```python
from build123d import *

# Parameters (mm, degrees)
SKETCH2_W           = 60
SKETCH2_H           = 32.5
BOSS_EXTRUDE1_DEPTH = 3
SKETCH3_W           = 8
SKETCH3_H           = 4
BOSS_EXTRUDE2_DEPTH = 13
FILLET1_R           = 3
SKETCH4_R           = 2.5
CUT_EXTRUDE1_DEPTH  = 13
SKETCH5_R           = 2.5
CUT_EXTRUDE2_DEPTH  = 13
FILLET2_R           = 3
BOSS_EXTRUDE3_DEPTH = 6.5
FILLET3_R           = 2
SKETCH7_W           = 40
SKETCH7_H           = 10
BOSS_EXTRUDE4_DEPTH = 30
CUT_EXTRUDE3_DEPTH  = 30
FILLET5_R           = 3
SKETCH9_R           = 1
CUT_EXTRUDE4_DEPTH  = 5
FILLET6_R           = 3
FILLET7_R           = 3
FILLET8_R           = 3


with BuildPart() as part:
    # Sketch2 → Boss-Extrude1 (new body)
    with BuildSketch(Plane.XY):
        with Locations((-25.634473236, 6.404480792)):
            Rectangle(SKETCH2_W, SKETCH2_H)
    extrude(amount=BOSS_EXTRUDE1_DEPTH)

    # Sketch3 → Boss-Extrude2 (add)
    with BuildSketch(Plane.XY.offset(3)):
        with Locations((0.365526764, 20.654480792)):
            Rectangle(SKETCH3_W, SKETCH3_H)
        with Locations((0.365526764, -7.845519208)):
            Rectangle(SKETCH3_W, SKETCH3_H)
        with Locations((-51.634473236, 20.654480792)):
            Rectangle(SKETCH3_W, SKETCH3_H)
        with Locations((-51.634473236, -7.845519208)):
            Rectangle(SKETCH3_W, SKETCH3_H)
    extrude(amount=BOSS_EXTRUDE2_DEPTH)

    # Fillet1
    fillet1_edges = [part.edges().sort_by_distance(p)[0] for p in [
        (4.365526764, 20.654480792, 16),
        (-3.634473236, 20.654480792, 16),
        (4.365526764, -7.845519208, 16),
        (-3.634473236, -7.845519208, 16),
        (-55.634473236, 20.654480792, 16),
        (-47.634473236, 20.654480792, 16),
        (-55.634473236, -7.845519208, 16),
        (-47.634473236, -7.845519208, 16),
    ]]
    fillet(fillet1_edges, radius=FILLET1_R)

    # Sketch4 → Cut-Extrude1 (cut)
    with BuildSketch(Plane(origin=(0, 22.654480792, 0), x_dir=(1, 0, 0), z_dir=(0, 1, 0))):
        with Locations(Location((0.365526764, -12, 0), (0, 0, 270))):
            Circle(SKETCH4_R)
        with Locations(Location((-51.634473236, -12, 0), (0, 0, 270))):
            Circle(SKETCH4_R)
    extrude(amount=-CUT_EXTRUDE1_DEPTH, mode=Mode.SUBTRACT)

    # Sketch5 → Cut-Extrude2 (cut)
    with BuildSketch(Plane(origin=(0, -5.845519208, 0), x_dir=(1, 0, 0), z_dir=(0, 1, 0))):
        with Locations(Location((-51.634473236, -12, 0), (0, 0, 270))):
            Circle(SKETCH5_R)
        with Locations(Location((0.365526764, -12, 0), (0, 0, 270))):
            Circle(SKETCH5_R)
    extrude(amount=-CUT_EXTRUDE2_DEPTH, mode=Mode.SUBTRACT)

    # Fillet2
    fillet2_edges = [part.edges().sort_by_distance(p)[0] for p in [
        (-3.634473236, 20.654480792, 3),
        (0.365526764, 18.654480792, 3),
        (0.365526764, -5.845519208, 3),
        (-3.634473236, -7.845519208, 3),
        (-51.634473236, 18.654480792, 3),
        (-47.634473236, 20.654480792, 3),
        (-47.634473236, -7.845519208, 3),
        (-51.634473236, -5.845519208, 3),
    ]]
    fillet(fillet2_edges, radius=FILLET2_R)

    # Sketch6 → Boss-Extrude3 (add)
    with BuildSketch(Plane.XY.offset(3)):
        with BuildLine():
            Line((-44.134473236, 7.654480792), (-7.134473236, 7.654480792))
            ThreePointArc((-7.134473236, 7.654480792), (-5.634473236, 6.154480792), (-7.134473236, 4.654480792))
            Line((-7.134473236, 4.654480792), (-44.134473236, 4.654480792))
            ThreePointArc((-44.134473236, 4.654480792), (-45.634473236, 6.154480792), (-44.134473236, 7.654480792))
        make_face()
    extrude(amount=BOSS_EXTRUDE3_DEPTH)

    # Fillet3
    fillet3_edges = [part.edges().sort_by_distance(p)[0] for p in [
        (-45.634473236, 6.154480792, 3),
        (-25.634473236, 4.654480792, 3),
        (-5.634473236, 6.154480792, 3),
        (-25.634473236, 7.654480792, 3),
    ]]
    fillet(fillet3_edges, radius=FILLET3_R)

    # Sketch7 → Boss-Extrude4 (add)
    with BuildSketch(Plane(origin=(0, 0, 0), x_dir=(-1, 0, 0), z_dir=(0, 0, -1))):
        with Locations((25.634473236, 6.404480792)):
            Rectangle(SKETCH7_W, SKETCH7_H)
    extrude(amount=BOSS_EXTRUDE4_DEPTH)

    # Sketch8 → Cut-Extrude3 (cut)
    with BuildSketch(Plane(origin=(0, 11.404480792, 0), x_dir=(1, 0, 0), z_dir=(0, 1, 0))):
        Polygon((-10.634473236, 10.954417446), (-13.99795844, 14.31790265), (-26.284293259, 3.42037636), (-37.226403791, 14.362486892), (-40.634473236, 10.954417446), (-40.634473236, 25.339784932), (-10.634473236, 25.339784932), align=None)
    extrude(amount=-CUT_EXTRUDE3_DEPTH, mode=Mode.SUBTRACT)

    # Fillet5
    fillet5_edges = [part.edges().sort_by_distance(p)[0] for p in [
        (-10.634473236, 6.404480792, -25.339784932),
        (-40.634473236, 6.404480792, -25.339784932),
    ]]
    fillet(fillet5_edges, radius=FILLET5_R)

    # Sketch9 → Cut-Extrude4 (cut)
    with BuildSketch(Plane(origin=(0, 0, -30), x_dir=(-1, 0, 0), z_dir=(0, 0, -1))):
        with Locations((26.284293259, 6.404480792)):
            Circle(SKETCH9_R)
    extrude(amount=-CUT_EXTRUDE4_DEPTH, mode=Mode.SUBTRACT)

    # Fillet6
    fillet6_edges = [part.edges().sort_by_distance(p)[0] for p in [
        (-13.99795844, 6.404480792, -14.31790265),
        (-26.284293259, 6.404480792, -3.42037636),
        (-37.226403791, 6.404480792, -14.362486892),
    ]]
    fillet(fillet6_edges, radius=FILLET6_R)

    # Fillet7
    fillet7_edges = [part.edges().sort_by_distance(p)[0] for p in [
        (-45.634473236, 6.404480792, 0),
        (-25.634473236, 11.404480792, 0),
        (-5.634473236, 6.404480792, 0),
        (-25.634473236, 1.404480792, 0),
    ]]
    fillet(fillet7_edges, radius=FILLET7_R)

    # Fillet8
    fillet8_edges = [part.edges().sort_by_distance(p)[0] for p in [
        (-45.634473236, 6.404480792, -30),
        (-5.634473236, 6.404480792, -30),
    ]]
    fillet(fillet8_edges, radius=FILLET8_R)


solid = part.part
```
The model under review builds one solid part; all positions refer to its coordinate system, in mm. A direction names the side the tool comes from. Round coordinates to 2 decimals unless told otherwise and drop trailing zeros. Loops run counter-clockwise (first coordinate to the right, second up) from the corner with the lowest first, then second, coordinate; pieces in that order, holes last. Notation, with made-up numbers: M 5,-19.75 L 61,-19.75 A14 ccw 61,-8.75 Z; hole C -1.5,58.5 d4. An arc over 180 degrees is marked long. Put each result on its own line as item: value.
Q1. Mouldability with a two-part tool opening along X and no side actions: class faces 4 (the flat face through (-25, 8, -30)), 5 (the cylindrical face through (-25.547, 7.08, -27.703)), 6 (the cylindrical face through (-46.941, 6.516, -0.524)) as released by +X, released by -X, zero draft, split by the parting line, or undercut.
Result set:
face 4: zero draft
face 5: undercut
face 6: released by -X
Q2. For pin 1 (1.3 mm diameter, centred on x = -20.5, z = 7.5, fed in from -Y); pin 2 (1.5 mm diameter, centred on x = -32.5, y = 9, fed in from +Z); pin 3 (4 mm diameter, centred on x = 0.37, z = 12, fed in from -Y); pin 4 (2.5 mm diameter, centred on x = -24, y = 5.5, fed in from +Z), all flat-tipped, find the tip position at first contact; note any pin that passes through.
Result set:
pin 1: stops at y = 4.65
pin 2: stops at z = 3.58
pin 3: passes through
pin 4: stops at z = 9.5
Q3. Machinability: for faces 1 (the cylindrical face through (-51.28, 17.752, 3.855)), 2 (the flat face through (-40.634, 6, -17)), 3 (the flat face through (-26, 7.654, 7)), which of the approach directions +Z, -Z, +X, -X, +Y, -Y give a long, thin tool a straight path to every point of the face, cutting with its end or side? Answer none if there is none.
Result set:
face 1: +Z, +X, -X
face 2: +Y, -Y
face 3: +Z, +X, -X, +Y
Q4. To check wall thickness, follow L1, parallel to Y at x = -53, z = 7.5; L2, parallel to X at y = 21, z = 12; L3, parallel to X at y = 7, z = -24. State the ranges of each line that lie inside material, in increasing order.
Result set:
L1: y = -9.85 to -5.85, 18.65 to 22.65
L2: x = -55.63 to -54.13, -49.13 to -47.63, -3.63 to -2.13, 2.87 to 4.37
L3: x = -45.63 to -40.13, -11.14 to -5.63
Q5. Consider section A-A, the plane z = 12. Count the separate pieces of the cut face and the enclosed holes in it, then the cut area to 3 significant figures.
Result set:
separate pieces: 8
enclosed holes: 0
area: 48.0 mm²
Q6. Consider section B-B, the plane x = -31. Give the boundary of the cut face in (y, z).
Result set:
outline: M -9.85,0 L -1.6,0 A3 cw 1.4,-3 L 1.4,-8.14 L 11.4,-8.14 L 11.4,-3 A3 cw 14.4,0 L 22.65,0 L 22.65,3 L 9.65,3 A2 cw 7.65,5 L 7.65,9.5 L 4.65,9.5 L 4.65,5 A2 cw 2.65,3 L -9.85,3 Z; M 1.4,-30 L 11.4,-30 L 11.4,-25.34 L 1.4,-25.34 Z
Q7. Consider section C-C, the plane z = -26. Give the boundary of the cut face in (x, y), then the cut area to 3 significant figures.
Result set:
outline: M -45.63,1.4 L -5.63,1.4 L -5.63,11.4 L -45.63,11.4 Z; hole C -26.28,6.4 d2
area: 397 mm²
